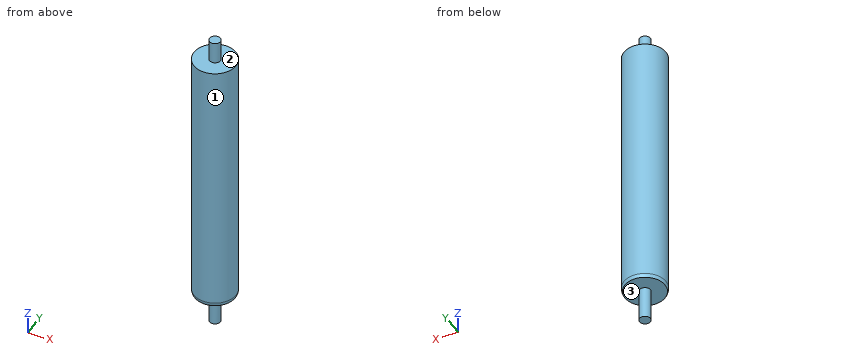
Autodesk Inventor part; units mm, degrees
ref_plane "YZ Plane" through (0, 0, 0) normal (1, 0, 0) x (0, 1, 0)
ref_plane "XZ Plane" through (0, 0, 0) normal (0, 1, 0) x (-1, 0, 0)
ref_plane "XY Plane" through (0, 0, 0) normal (0, 0, 1) x (1, 0, 0)
sketch "Sketch1" plane through (0, 0, 0) normal (0, 0, 1) x (1, 0, 0)
  circle A0 centre (0, 0) radius 5.78
  dimension "d0" = 11.56
extrude "Extrusion1" add sketch "Sketch1" along normal blind 80
fillet "Fillet1" radius 2 2 edges at (-5.78, 0, 80) (-5.78, 0, 0)
sketch "Sketch2" plane through (0, 0, 80) normal (0, 0, 1) x (1, 0, 0)
  circle A0 centre (0, 0) radius 1.5
  circle A1 centre (0, 0) radius 5.78
  dimension "d4" = 3
  dimension "d5" = 11.56
extrude "Extrusion2" cut sketch "Sketch2" against normal blind 6
sketch "Sketch3" plane through (0, 0, 0) normal (0, 0, -1) x (-1, 0, 0)
  circle A0 centre (0, 0) radius 1.5
  circle A1 centre (0, 0) radius 1.5
  circle A2 centre (0, 0) radius 5.78
extrude "Extrusion3" cut sketch "Sketch3" against normal blind 1
sketch "Sketch4" plane through (0, 0, 0) normal (0, 0, -1) x (-1, 0, 0)
  circle A0 centre (0, 0) radius 1.5
extrude "Extrusion4" add sketch "Sketch4" along normal blind 8
properties part number "cylinder"
Geometry check sheet. Reference: the model listing, model coordinates, mm. Face numbers are marked on the shaded views. A direction names the side the tool comes from. Give positions to 0.01 mm unless a question says otherwise; leave off trailing zeros. Loops run counter-clockwise (first coordinate to the right, second up) from the corner with the lowest first, then second, coordinate; pieces in that order, holes last. Notation, with made-up numbers: (75.5, 31.25) -> (129.5, 31.25) arc R29 cw to (129.5, 67.25) -> close; hole circle Ø4 at (74, 85). An arc over 180 degrees is marked (long way). Answer in a Markdown table with one row per item. Add a question column.
1) Material ranges on probe 1 along Y at (x, z) = (-0.25, 27); probe 2 along Z at (x, y) = (1.25, -3.5); probe 3 along Y at (x, z) = (2, 11.5), recorded low to high. Write a range as from..to.
2) Cross-section at A-A on x = 0. Record the boundary of the cut face in (y, z), and give its area (3 significant figures).
3) Set-up check for the marked faces 1, 2 and 3: record each of +Z, -Z, +X, -X, +Y, -Y from which the full face is reachable in a straight line by a thin tool's end or side.
4) Cross-section at C-C on z = 59. Record the boundary of the cut face in (x, y), and give its area (3 significant figures).
5) Gauge pin test, flat ends, axial feed: P1, Ø3, axis at y = 1, z = 5.5, coming from the +X side; P2, Ø2, axis at y = 3.5, z = 3.5, coming from the -X side; P3, Ø4, axis at y = 3.5, z = 24, coming from the -X side; P4, Ø1.5, axis at y = -2.5, z = 33, coming from the -X side. Record the tip position at first contact, or that the pin passes through.
Outcome:
| question | item | result |
|---|---|---|
| 1 | probe 1 | y = -5.77..5.77 |
| 1 | probe 2 | z = 1..74 |
| 1 | probe 3 | y = -5.42..5.42 |
| 2 | outline | (-5.78, 2) arc R2 ccw to (-5.51, 1) -> (-1.5, 1) -> (-1.5, -8) -> (1.5, -8) -> (1.5, 1) -> (5.51, 1) arc R2 ccw to (5.78, 2) -> (5.78, 74) -> (1.5, 74) -> (1.5, 80) -> (-1.5, 80) -> (-1.5, 74) -> (-5.78, 74) -> close |
| 2 | area | 889 mm^2 |
| 3 | face 1 | +Z, -Z |
| 3 | face 2 | +Z |
| 3 | face 3 | -Z |
| 4 | outline | circle Ø11.56 at (0, 0) |
| 4 | area | 105 mm^2 |
| 5 | P1 | stops at x = 5.78 |
| 5 | P2 | stops at x = -5.21 |
| 5 | P3 | stops at x = -5.58 |
| 5 | P4 | stops at x = -5.51 |
